Input: part model. Units: mm. Frame: model coordinates. A direction names the side the tool comes from. Coordinates: 2 decimals unless noted, no trailing zeros. Loops run counter-clockwise (first coordinate to the right, second up) from the corner with the lowest first, then second, coordinate; pieces in that order, holes last. Notation, with made-up numbers: M 47,-20 L 96,-20 A31 cw 96,11 Z; hole C -34.75,-15 d1. An arc over 180 degrees is marked long. Use a Markdown table: item, result. Add a question column.
1. Line query: L1, parallel to Y at x = -8.5, z = -15; L2, parallel to X at y = 46, z = 0.25; L3, parallel to Z at x = -19, y = 48.5. Output: solid intervals per line, ascending. Write a range as [from, to].
2. Draft query along Y for faces 4 (the flat face through (-3, 16.835, -12)), 5 (the flat face through (-3, 46.835, 1)), 6 (the flat face through (-3, 16, -24)). Return one class per face: +Y half, -Y half, draft (parallel to the pull), parting line (faces both ways), or undercut.
3. Section B-B on y = 46. Output: boundary loops of the cut face in (x, z).
4. Section A-A on x = -18. Output: boundary loops of the cut face in (y, z).
5. Pin query (flat end, axial travel): pin 1 (8 mm diameter, centred on x = 15, z = -20, fed in from +Y); pin 2 (12 mm diameter, centred on y = 38.5, z = -6.5, fed in from +X); pin 3 (8 mm diameter, centred on y = 37, z = -3, fed in from -X). Return the tip coordinate at first contact, or that it passes through.
6. Section D-D on y = 20. Output: boundary loops of the cut face in (x, z).
7. Set-up query: faces 1 (the flat face through (20.216, 34, 1)), 2 (the flat face through (-3, 50.835, 1)), 3 (the flat face through (-2, 49, 0)). Return all of +Z, -Z, +X, -X, +Y, -Y with unobstructed straight access to the full face (end or side cutting, diameter ignored); none if empty.
```python
from build123d import *

# Parameters (mm, degrees)
SKETCH1_W           = 53
SKETCH1_H           = 2
SKETCH1_H_2         = 34
SKETCH1_W_2         = 45
SKETCH1_H_3         = 26
BOSS_EXTRUDE1_DEPTH = 2
SKETCH1_5_W         = 53
SKETCH1_5_H         = 2
BOSS_EXTRUDE4_DEPTH = 24
FILLET2_R           = 1


with BuildPart() as part:
    # Sketch1 → Boss-Extrude1 (new body)
    # profile 1 of 2: a face of its own
    with BuildSketch(Plane.XY):
        with Locations((-2.283686935, 15.83542926)):
            Rectangle(SKETCH1_W, SKETCH1_H)
    # profile 2 of 2: a face of its own
    with BuildSketch(Plane.XY):
        with Locations((-2.283686935, 33.83542926)):
            Rectangle(SKETCH1_W, SKETCH1_H_2)
        with Locations((-2.283686935, 33.83542926)):
            Rectangle(SKETCH1_W_2, SKETCH1_H_3, mode=Mode.SUBTRACT)
    extrude(amount=BOSS_EXTRUDE1_DEPTH)

    # Sketch1<5> → Boss-Extrude4 (add)
    with BuildSketch(Plane.XY):
        with Locations((-2.283686935, 15.83542926)):
            Rectangle(SKETCH1_5_W, SKETCH1_5_H)
    extrude(amount=-BOSS_EXTRUDE4_DEPTH)

    # Fillet2
    fillet2_edges = [part.edges().sort_by_distance(p)[0] for p in [
        (-28.783686935, 33.83542926, 0),
        (24.216313065, 33.83542926, 0),
        (-2.283686935, 16.83542926, 0),
        (-28.783686935, 16.83542926, -12),
        (24.216313065, 16.83542926, -12),
        (24.216313065, 50.83542926, 1),
        (24.216313065, 14.83542926, -11),
        (-28.783686935, 50.83542926, 1),
        (-28.783686935, 14.83542926, -11),
    ]]
    fillet(fillet2_edges, radius=FILLET2_R - 0.0001)  # a hair under: the kernel refuses the full size


solid = part.part
```
Answers below:
| question | item | result |
|---|---|---|
| 1 | L1 | y = [14.84, 16.84] |
| 1 | L2 | x = [-28.45, -24.78], [20.22, 23.88] |
| 1 | L3 | z = [0, 2] |
| 2 | face 4 | +Y half |
| 2 | face 5 | undercut |
| 2 | face 6 | draft |
| 3 | outline | M -28.78,1 A1 ccw -27.78,0 L -24.78,0 L -24.78,2 L -28.78,2 Z; M 20.22,0 L 23.22,0 A1 ccw 24.22,1 L 24.22,2 L 20.22,2 Z |
| 4 | outline | M 14.84,-24 L 16.84,-24 L 16.84,-1 A1 cw 17.84,0 L 20.84,0 L 20.84,2 L 14.84,2 Z; M 46.84,0 L 50.84,0 L 50.84,2 L 46.84,2 Z |
| 5 | pin 1 | stops at y = 16.84 |
| 5 | pin 2 | passes through |
| 5 | pin 3 | stops at x = -28.78 |
| 6 | outline | M -28.78,1 A1 ccw -27.78,0 L 23.22,0 A1 ccw 24.22,1 L 24.22,2 L -28.78,2 Z |
| 7 | face 1 | +Z, -Z |
| 7 | face 2 | +Z, -Z, +X, -X, +Y |
| 7 | face 3 | -Z, +X, -X, +Y |
